CAD build for the part. Positions are in the model's coordinates, mm. A direction names the side the tool comes from. Round coordinates to 2 decimals unless told otherwise and drop trailing zeros. Loops run counter-clockwise (first coordinate to the right, second up) from the corner with the lowest first, then second, coordinate; pieces in that order, holes last. Notation, with made-up numbers: (84.25, 36) - (130.25, 36) arc R11 ccw to (130.25, 47) - close; hole circle Ø2 at (65, -19.5). An arc over 180 degrees is marked (long way). One line per question, with ' | ' between items.
```python
from build123d import *

# Parameters (mm, degrees)
F0_W     = 55.675162
F0_H     = 14.010968
F1_DEPTH = 5.08
F2_R     = 1.739199
F2_R_2   = 1.342124
F3_DEPTH = 101.6
F4_R     = 1.704997
F5_DEPTH = 25.4


with BuildPart() as f1:
    # F0 (on Front) → F1 (new body)
    with BuildSketch(Plane.XZ):
        with Locations((14.103145, 12.075242)):
            Rectangle(F0_W, F0_H)
    extrude(amount=F1_DEPTH)

    # F2 (on face) → F3 (join)
    with BuildSketch(Plane.XY.offset(19.080726)):
        with Locations((14.103145, -2.48879)):
            Circle(F2_R)
        with Locations((14.103145, -2.48879)):
            Circle(F2_R_2, mode=Mode.SUBTRACT)
    extrude(amount=-F3_DEPTH)

    # F4 (on face) → F5 (cut)
    with BuildSketch(Plane.XY.offset(19.080726)):
        with Locations((14.103145, -2.971026)):
            Circle(F4_R)
    extrude(amount=-F5_DEPTH, mode=Mode.SUBTRACT)


solid = f1.part
```
(1) Cut at C-C, the plane z = -60.5. Write the cut outline in (x, y), then the cut area to 3 significant figures.
Results found:
outline: circle Ø3.48 at (14.1, -2.49); hole circle Ø2.68 at (14.1, -2.49) | area: 3.84 mm²
(2) Drop flat-ended pins along their axis: P1, Ø10, axis at x = 10, z = -38, coming from the -Y side; P2, Ø1, axis at x = 19, y = -4, coming from the -Z side; P3, Ø3, axis at x = 14, y = -3, coming from the +Z side. Give the stop position or say it passes through.
Results found:
P1: stops at y = -4.23 | P2: stops at z = 5.07 | P3: stops at z = -6.32
(3) Cut at B-B, the plane z = 6.5. Write the cut outline in (x, y) (3 decimals), then the cut area to 3 significant figures.
Results found:
outline: (-13.734, -5.08) - (41.941, -5.08) - (41.941, 0) - (-13.734, 0) - close; hole circle Ø3.41 at (14.103, -2.971) | area: 274 mm²
(4) Two-plate mould, pull along X, no slides. Class faces 1 (the face through (14, -4, -6.319)), 2 (the face through (13.877, -0.764, -38.112)), 3 (the face through (-13.734, -3, 12)), 4 (the face through (14, -1, 19.081)): released by +X, released by -X, zero draft, split by the parting line, or undercut.
Results found:
face 1: undercut | face 2: split by the parting line | face 3: released by -X | face 4: zero draft
(5) Probe L1, parallel to X at y = -2.7, z = -42; L2, parallel to Z at x = -2, y = -4.15; L3, parallel to X at y = -3.45, z = -28. List the from-to ranges inside material, lowest first.
Results found:
L1: x = 12.38 to 12.78, 15.43 to 15.83 | L2: z = 5.07 to 19.08 | L3: x = 12.65 to 13.17, 15.04 to 15.55
(6) Tool access for faces 5 (the face through (13.928, -1.158, -38.112)), 6 (the face through (13.88, -1.28, 9.38)), 7 (the face through (41.941, -3, 12)): list every direction of +Z, -Z, +X, -X, +Y, -Y with a clear straight run to the whole face (end or side of a thin tool).
Results found:
face 5: -Z | face 6: +Z | face 7: +Z, -Z, +X, +Y, -Y
(7) Cut at A-A, the plane x = 29. Write the cut outline in (y, z).
Results found:
outline: (-5.08, 5.07) - (0, 5.07) - (0, 19.08) - (-5.08, 19.08) - close
